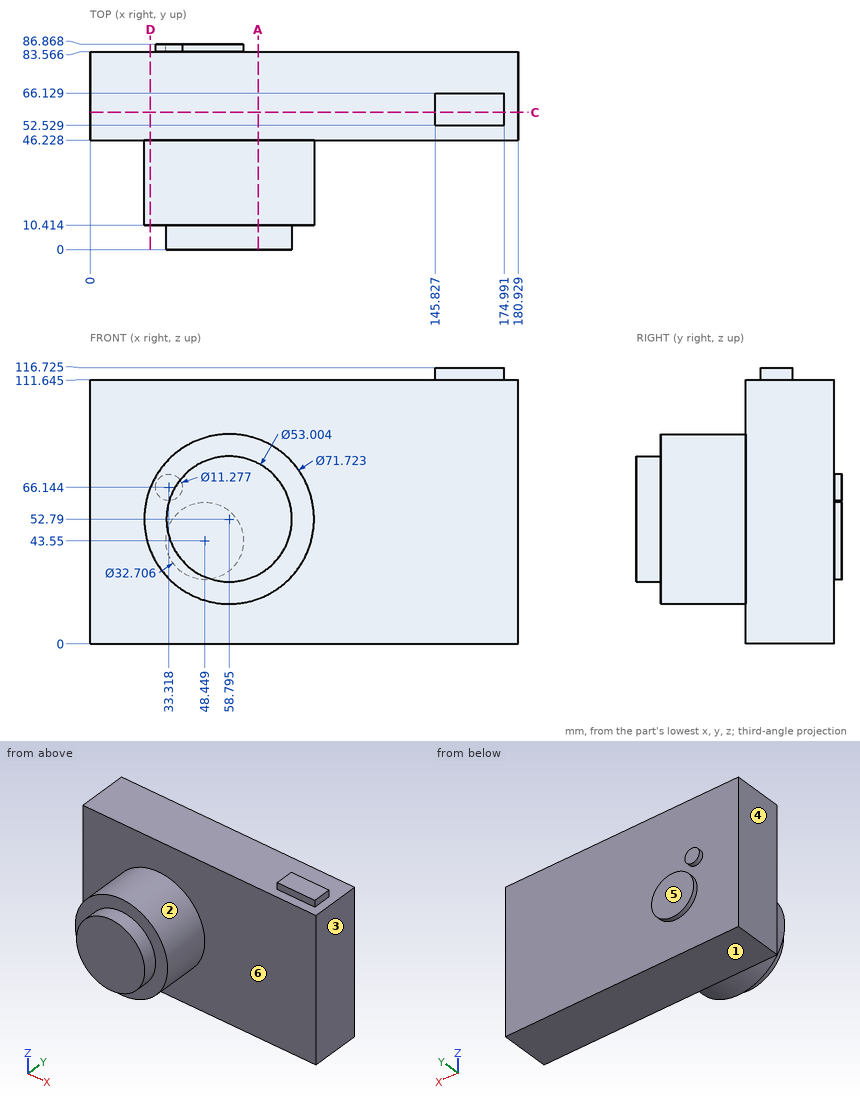
The drawing under review shows one solid part. Ordinate dimensions are in mm from its lowest x, y, z. A direction names the side the tool comes from. Give positions to 0.01 mm unless a question says otherwise; leave off trailing zeros. Loops run counter-clockwise (first coordinate to the right, second up) from the corner with the lowest first, then second, coordinate; pieces in that order, holes last. Notation, with made-up numbers: M -38.75,83.5 L -29.75,83.5 A28 ccw -29.75,120.5 Z; hole C 48,70 d11. An arc over 180 degrees is marked long. One line per question, with ' | ' between items. Start each with the question number.
1. The part is to be moulded in two halves that separate along X. For the marked faces 1, 2, 3 and 4, say which applies: released by +X, released by -X, zero draft, split by the parting line, or undercut.
2. Add section C-C (y = 58). Write out the cut boundary in (x, z) (1 decimal).
3. Add section D-D (x = 25.5). Write out the cut boundary in (y, z) (1 decimal).
4. For the marked faces 5 and 6, list the 3-axis set-ups (+Z, -Z, +X, -X, +Y, -Y) from which the entire face can be reached by the end or side of a thin tool; tool diameter is ignored.
5. Insertion check: P1, Ø1, axis at x = 102.5, z = 31.5, coming from the +Y side; P2, Ø11, axis at x = 92.5, y = 65, coming from the +Z side (1 decimal); P3, Ø1.5, axis at y = 56.5, z = 115, coming from the -X side; P4, Ø5.5, axis at y = 57.5, z = 113.5, coming from the +X side. Each pin has a flat end and moves straight along its axis. Give the tip position at first contact, or say it passes through.
6. Add section A-A (x = 71). Write out the cut boundary in (y, z) (1 decimal).
7. To check wall thickness, follow L1, parallel to Y at x = 94, z = 50.5 (1 decimal); L2, parallel to Y at x = 162, z = 109.5 (1 decimal); L3, parallel to Z at x = 97.5, y = 67 (1 decimal). State the ranges of each line that lie inside material, in increasing order.
Worked out:
1) face 1: zero draft | face 2: split by the parting line | face 3: released by +X | face 4: released by -X
2) outline: M 0,0 L 180.9,0 L 180.9,111.6 L 175,111.6 L 175,116.7 L 145.8,116.7 L 145.8,111.6 L 0,111.6 Z
3) outline: M 10.4,39.5 L 46.2,39.5 L 46.2,0 L 83.6,0 L 83.6,111.6 L 46.2,111.6 L 46.2,66.1 L 10.4,66.1 Z
4) face 5: +Z, -Z, +X, -X, +Y | face 6: -Y
5) P1: stops at y = 83.57 | P2: stops at z = 111.6 | P3: stops at x = 145.83 | P4: stops at x = 180.93
6) outline: M 0,29.3 L 10.4,29.3 L 10.4,19.1 L 46.2,19.1 L 46.2,0 L 83.6,0 L 83.6,111.6 L 46.2,111.6 L 46.2,86.5 L 10.4,86.5 L 10.4,76.3 L 0,76.3 Z
7) L1: y = 10.4 to 83.6 | L2: y = 46.2 to 83.6 | L3: z = 0 to 111.6
